Work out the finished part from the listing and answer in its coordinate system (mm). A direction names the side the tool comes from. Coordinates: 2 decimals unless noted, no trailing zeros. Write each loop counter-clockwise with the first axis right and the second up, starting at its lowest first coordinate (ties: lowest second). Pieces come first, ordered by that corner, then holes. Notation, with made-up numbers: (69.5, 72) -> (111.5, 72) arc R15 ccw to (111.5, 89) -> close; hole circle Ø9 at (-35.75, 42.5). An arc over 180 degrees is marked (long way). Write each question's results on one line, items separated by ' | '. Start each with the question number.
from build123d import *

# Parameters (mm, degrees)
AUFSATZ_LINEAR_AUSTRAGEN2_DEPTH                = 13
STIRNSENKUNG_START                             = 26.95
STIRNSENKUNG_LANGLOCH_F_R_M4_FLACHKOPFSC_DEPTH = 3.1
STIRNSENKUNG_START_2                           = 25.05
STIRNSENKUNG_LANGLOCH_F_R_M4_FLACHKO_3_DEPTH   = 1.9
SCHNITT_LINEAR_AUSTRAGEN1_DEPTH                = 91.954672777
SCHNITT_LINEAR_AUSTRAGEN1_DEPTH_BACK           = 91.954672777
VERRUNDUNG1_R                                  = 10
AUFSATZ_LINEAR_AUSTRAGEN4_REACH                = 65.751
SKIZZE9_W                                      = 3
SKIZZE9_H                                      = 26.5
AUFSATZ_LINEAR_AUSTRAGEN4_DIRECTION_2_REACH    = 65.751
SKIZZE18_W                                     = 110
SKIZZE18_H                                     = 4.5
AUFSATZ_LINEAR_AUSTRAGEN5_DEPTH                = 2
F_4_2_4_2_DURCHMESSER_BOHRUNG1_D               = 4.2
SKIZZE19_R                                     = 6.5
SCHNITT_LINEAR_AUSTRAGEN2_DEPTH                = 11
M5_GEWINDEBOHRUNG1_REACH                       = 73.925
M5_GEWINDEBOHRUNG1_BORE_R                      = 2.1
VERRUNDUNG2_R                                  = 2


# Read off the part's stored shape, not the designer's step: Stirnsenkung Langloch für M4 Flachkopfschraube mit Schlitz12
with BuildPart() as part:
    # Skizze2 → Aufsatz-Linear austragen2 (new, symmetric)
    with BuildSketch(Plane.XY):
        Polygon((-25.05, -25), (-25.05, 0), (25.05, 0), (25.05, -25), (30.05, -25), (30.05, 0), (55, 0), (55, 29.5), (-55, 29.5), (-55, 0), (-30.05, 0), (-30.05, -25), align=None)
    extrude(amount=AUFSATZ_LINEAR_AUSTRAGEN2_DEPTH, both=True)

    # Stirnsenkung Langloch f_r M4 Flachko 2 → Stirnsenkung Langloch für M4 Flachkopfschraube mit Schlitz12 (cut)
    with BuildSketch(Plane.YZ.offset(STIRNSENKUNG_START)):
        with BuildLine():
            Line((-5.25, -1.5), (-18.75, -1.5))
            ThreePointArc((-18.75, -1.5), (-23.25, -6), (-18.75, -10.5))
            Line((-18.75, -10.5), (-5.25, -10.5))
            ThreePointArc((-5.25, -10.5), (-0.75, -6), (-5.25, -1.5))
        make_face()
    stirnsenkung_langloch_f_r_m4_flachkopfsc = extrude(amount=STIRNSENKUNG_LANGLOCH_F_R_M4_FLACHKOPFSC_DEPTH, mode=Mode.SUBTRACT)

    # Stirnsenkung Langloch f_r M4 Flachko 3 o → Stirnsenkung Langloch f_r M4 Flachko 3 (cut)
    with BuildSketch(Plane.YZ.offset(STIRNSENKUNG_START_2)):
        with BuildLine():
            Line((-5.25, -3.75), (-18.75, -3.75))
            ThreePointArc((-18.75, -3.75), (-21, -6), (-18.75, -8.25))
            Line((-18.75, -8.25), (-5.25, -8.25))
            ThreePointArc((-5.25, -8.25), (-3, -6), (-5.25, -3.75))
        make_face()
    stirnsenkung_langloch_f_r_m4_flachko_3 = extrude(amount=STIRNSENKUNG_LANGLOCH_F_R_M4_FLACHKO_3_DEPTH, mode=Mode.SUBTRACT)

    # Skizze5 → Schnitt-Linear austragen1 (cut, two sides: drawn at the far end of the back side and taken through both)
    with BuildSketch(Plane(origin=(30.05, 0, 0), x_dir=(0, 0, -1), z_dir=(1, 0, 0)).offset(-SCHNITT_LINEAR_AUSTRAGEN1_DEPTH_BACK)):
        Polygon((-10, 0), (-10, 25), (-13, 25), (-13, -25), (-5, -25), (-5, 0), align=None)
    extrude(amount=SCHNITT_LINEAR_AUSTRAGEN1_DEPTH + SCHNITT_LINEAR_AUSTRAGEN1_DEPTH_BACK, mode=Mode.SUBTRACT)

    # Verrundung1
    # the kernel refuses this fillet: 10 mm, written as the material it adds along each edge
    with BuildSketch(Plane(origin=(-25.05, 0, 5), x_dir=(0, 0, 1), z_dir=(-1, 0, 0))) as verrundung1_piece_1:
        with BuildLine():
            CenterArc((10, -8.660254038), VERRUNDUNG1_R, 120, 60)
            Line((0, -8.660254038), (-0.2, -8.660254038))
            Line((-0.2, -8.660254038), (-0.2, 0))
            Line((-0.2, 0), (0, 0.2))
            ThreePointArc((0, 0.2), (2.5, 0.2), (4.9, 0.173205081))
            Line((4.9, 0.173205081), (5, 0))
        make_face()
    extrude(amount=5)
    with BuildSketch(Plane(origin=(30.05, 0, 5), x_dir=(0, -1, 0), z_dir=(-1, 0, 0))) as verrundung1_piece_2:
        with BuildLine():
            CenterArc((8.660254038, 10), VERRUNDUNG1_R, 210, 60)
            Line((0, 5), (-0.173205081, 4.9))
            ThreePointArc((-0.173205081, 4.9), (-0.2, 2.5), (-0.2, 0))
            Line((-0.2, 0), (0, -0.2))
            Line((0, -0.2), (8.660254038, -0.2))
            Line((8.660254038, -0.2), (8.660254038, 0))
        make_face()
    extrude(amount=5)

    # Aufsatz-Linear austragen4: up to this face of the body (flat: up to its plane)
    aufsatz_linear_austragen4_end = Plane(part.part.faces().sort_by_distance((55, 14.993858382, -1.246387283))[0])
    # Skizze9 → Aufsatz-Linear austragen4 (add, up to the picked face)
    with BuildSketch(Plane(origin=(0, 0, 0), x_dir=(0, 0, -1), z_dir=(1, 0, 0)), mode=Mode.PRIVATE) as aufsatz_linear_austragen4_sk1:
        with Locations((14.5, 16.25)):
            Rectangle(SKIZZE9_W, SKIZZE9_H)
    aufsatz_linear_austragen4_tool1 = split(extrude(aufsatz_linear_austragen4_sk1.sketch, amount=AUFSATZ_LINEAR_AUSTRAGEN4_REACH, mode=Mode.PRIVATE), bisect_by=aufsatz_linear_austragen4_end, keep=Keep.BOTH, mode=Mode.PRIVATE)
    add(aufsatz_linear_austragen4_tool1.solids().sort_by(Axis((0, 16.25, -14.5), (1, 0, 0)))[0])

    # Aufsatz-Linear austragen4 direction 2: up to this face of the body (flat: up to its plane)
    aufsatz_linear_austragen4_direction_2_end = Plane(part.part.faces().sort_by_distance((-55, 14.993858382, -1.246387283))[0])
    # Skizze9 → Aufsatz-Linear austragen4 direction 2 (add, up to the picked face)
    with BuildSketch(Plane(origin=(0, 0, 0), x_dir=(0, 0, -1), z_dir=(1, 0, 0)), mode=Mode.PRIVATE) as aufsatz_linear_austragen4_direction_2_sk1:
        with Locations((14.5, 16.25)):
            Rectangle(SKIZZE9_W, SKIZZE9_H)
    aufsatz_linear_austragen4_direction_2_tool1 = split(extrude(aufsatz_linear_austragen4_direction_2_sk1.sketch, amount=-AUFSATZ_LINEAR_AUSTRAGEN4_DIRECTION_2_REACH, mode=Mode.PRIVATE), bisect_by=aufsatz_linear_austragen4_direction_2_end, keep=Keep.BOTH, mode=Mode.PRIVATE)
    add(aufsatz_linear_austragen4_direction_2_tool1.solids().sort_by(Axis((0, 16.25, -14.5), (-1, 0, 0)))[0])

    # Skizze18 → Aufsatz-Linear austragen5 (add)
    with BuildSketch(Plane.XY.offset(13)):
        with Locations((0, 27.25)):
            Rectangle(SKIZZE18_W, SKIZZE18_H)
    extrude(amount=AUFSATZ_LINEAR_AUSTRAGEN5_DEPTH)

    # Ø4.2 (4.2) Durchmesser Bohrung1 (through all)
    with Locations(Plane(origin=(55, 0, 0), x_dir=(0, 0, -1), z_dir=(1, 0, 0))):
        with Locations((0, 5)):
            Hole(F_4_2_4_2_DURCHMESSER_BOHRUNG1_D / 2)

    # Spiegeln2: Stirnsenkung Langloch für M4 Flachkopfschraube mit Schlitz12, Stirnsenkung Langloch f_r M4 Flachko 3 across plane
    add(stirnsenkung_langloch_f_r_m4_flachkopfsc.mirror(Plane(origin=(0, 0, 0), x_dir=(0, 0, 1), z_dir=(1, 0, 0))), mode=Mode.SUBTRACT)
    add(stirnsenkung_langloch_f_r_m4_flachko_3.mirror(Plane(origin=(0, 0, 0), x_dir=(0, 0, 1), z_dir=(1, 0, 0))), mode=Mode.SUBTRACT)

    # Skizze19 → Schnitt-Linear austragen2 (cut)
    with BuildSketch(Plane(origin=(0, 29.5, 0), x_dir=(1, 0, 0), z_dir=(0, 1, 0))):
        with Locations(Location((-35, 0, 0), (0, 0, 270))):
            Circle(SKIZZE19_R)
        with Locations(Location((35, 0, 0), (0, 0, 90))):
            Circle(SKIZZE19_R)
    extrude(amount=-SCHNITT_LINEAR_AUSTRAGEN2_DEPTH, mode=Mode.SUBTRACT)

    # M5 Gewindebohrung1 bore → M5 Gewindebohrung1 (cut, up to next)
    with BuildSketch(Plane(origin=(0, 18.5, 0), x_dir=(1, 0, 0), z_dir=(0, 1, 0)), mode=Mode.PRIVATE) as m5_gewindebohrung1_sk1:
        with Locations((-35, 0)):
            Circle(M5_GEWINDEBOHRUNG1_BORE_R)
    m5_gewindebohrung1_tool1 = extrude(m5_gewindebohrung1_sk1.sketch, amount=-M5_GEWINDEBOHRUNG1_REACH, mode=Mode.PRIVATE) & part.part
    m5_gewindebohrung1 = m5_gewindebohrung1_tool1.solids().sort_by_distance((-35, 18.5, 0))[0]
    add(m5_gewindebohrung1, mode=Mode.SUBTRACT)

    # Verrundung2
    verrundung2_edges = [part.edges().sort_by_distance(p)[0] for p in [
        (-55, 27.25, 15),
        (0, 25, 15),
        (55, 27.25, 15),
        (55, 12.5, 10),
        (55, 25, 12.5),
        (-55, 25, 12.5),
        (0, 25, 10),
        (-55, 12.5, 10),
    ]]
    fillet(verrundung2_edges, radius=VERRUNDUNG2_R)

    # Spiegeln3: M5 Gewindebohrung1 across plane
    add(m5_gewindebohrung1.mirror(Plane(origin=(0, 0, 0), x_dir=(0, 0, 1), z_dir=(1, 0, 0))), mode=Mode.SUBTRACT)


solid = part.part
1. Find section A-A on y = -12.5. Give the vertices of the cut face in (x, z).
2. Given pin 1 Ø1.5 at (y, z) = (-2, 8) entering from -X; pin 2 Ø0.9 at (x, y) = (-28.5, -10) entering from +Z; pin 3 Ø7 at (x, z) = (39.5, 0) entering from -Y, each flat-ended and moving along its own axis, determine where each tip first touches the part or whether it passes through.
3. For faces 5 (the face through (28.48, -23.25, -5.9)), 6 (the face through (30.05, -13, -1)), 7 (the face through (-28.555, 24.077, -0.846)), determine the directions among +Z, -Z, +X, -X, +Y, -Y from which every point of the face is accessible in a straight line to the end or side of a thin tool.
4. Find section D-D on x = -35. Give the vertices of the cut face in (y, z), and give its area (3 significant figures).
5. Find the intervals of material crossed by L1, parallel to X at y = 24, z = 0; L2, parallel to X at y = 10.25, z = 0; L3, parallel to Z at x = 35, y = 11, in increasing order.
6. Find section C-C on z = 0. Give the number of separate pieces and of enclosed holes in the cut face, and give its area (3 significant figures).
7. Determine the mould class of faces 1 (the face through (28.555, 24.077, 0.846)), 2 (the face through (-26.95, -12, -9)), 3 (the face through (-28, -12, -1.5)), 4 (the face through (-43, 0, -1)) for opening direction Y: pulls with the +Y half, pulls with the -Y half, needs draft (parallel to the pull), parting line crosses it, or undercut.
8. Find section B-B on x = 2. Give the vertices of the cut face in (y, z), and give its area (3 significant figures).
Ans:
1) outline: (-30.05, -13) -> (-25.05, -13) -> (-25.05, -8.25) -> (-26.95, -8.25) -> (-26.95, -10.5) -> (-30.05, -10.5) -> close; (-30.05, -1.5) -> (-26.95, -1.5) -> (-26.95, -3.75) -> (-25.05, -3.75) -> (-25.05, 5) -> (-30.05, 5) -> close; (25.05, -13) -> (30.05, -13) -> (30.05, -10.5) -> (26.95, -10.5) -> (26.95, -8.25) -> (25.05, -8.25) -> close; (25.05, -3.75) -> (26.95, -3.75) -> (26.95, -1.5) -> (30.05, -1.5) -> (30.05, 5) -> (25.05, 5) -> close
2) pin 1: stops at x = -30.05 | pin 2: stops at z = 5 | pin 3: stops at y = 0
3) face 5: +X | face 6: +Z, -Z, +X, -Y | face 7: +Y
4) outline: (0, -13) -> (3, -13) -> (3, -16) -> (29.5, -16) -> (29.5, -6.5) -> (18.5, -6.5) -> (18.5, -2.1) -> (5, -2.1) arc R2.1 cw to (5, 2.1) -> (18.5, 2.1) -> (18.5, 6.5) -> (29.5, 6.5) -> (29.5, 15) -> (27, 15) arc R2 ccw to (25, 13) -> (25, 12) arc R2 cw to (23, 10) -> (0, 10) -> close | area: 574 mm²
5) L1: x = -55 to -41.5, -28.5 to 28.5, 41.5 to 55 | L2: x = -55 to -37.1, -32.9 to 32.9, 37.1 to 55 | L3: z = -16 to -2.1, 2.1 to 10
6) separate pieces: 4 | enclosed holes: 0 | area: 2,650 mm²
7) face 1: needs draft | face 2: undercut | face 3: undercut | face 4: pulls with the -Y half
8) outline: (0, -13) -> (3, -13) -> (3, -16) -> (29.5, -16) -> (29.5, 15) -> (27, 15) arc R2 ccw to (25, 13) -> (25, 12) arc R2 cw to (23, 10) -> (0, 10) -> close; hole circle Ø4.2 at (5, 0) | area: 767 mm²
